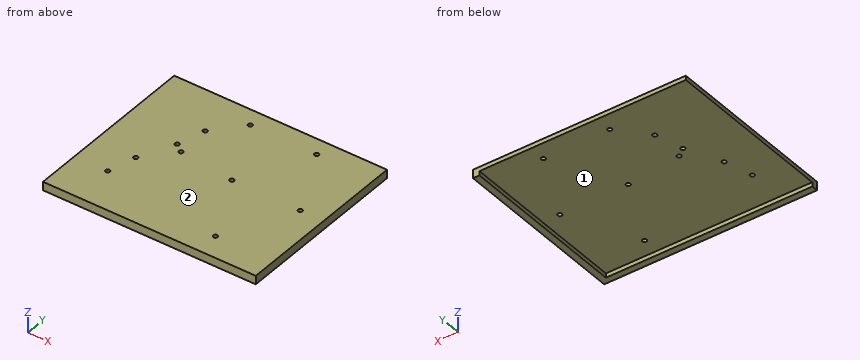
from build123d import *

# Parameters (mm, degrees)
F0_W     = 153.1874
F0_H     = 127
F0_R     = 1.5875
F1_DEPTH = 3.175
F2_DEPTH = 3.175


with BuildPart() as f1:
    # F0 (on Top) → F1 (new body)
    with BuildSketch(Plane.XY):
        Polygon((76.5937, 63.5), (76.5937, -63.5), (-76.5937, -63.5), (-76.5937, -68.2625), (81.3562, -68.2625), (81.3562, 63.5), align=None)
        Rectangle(F0_W, F0_H)
        with Locations((-51.98999, -36.501629)):
            Circle(F0_R, mode=Mode.SUBTRACT)
        with Locations((-46.4312, -15.875)):
            Circle(F0_R, mode=Mode.SUBTRACT)
        with Locations((38.4937, -50.8)):
            Circle(F0_R, mode=Mode.SUBTRACT)
        with Locations((-28.17241, 4.751629)):
            Circle(F0_R, mode=Mode.SUBTRACT)
        with Locations((-34.52749, 9.535871)):
            Circle(F0_R, mode=Mode.SUBTRACT)
        with Locations((-28.9687, 30.1625)):
            Circle(F0_R, mode=Mode.SUBTRACT)
        with Locations((-10.70991, 50.789129)):
            Circle(F0_R, mode=Mode.SUBTRACT)
        with Locations((13.0937, 0)):
            Circle(F0_R, mode=Mode.SUBTRACT)
        with Locations((63.8937, 0)):
            Circle(F0_R, mode=Mode.SUBTRACT)
        with Locations((38.4937, 50.8)):
            Circle(F0_R, mode=Mode.SUBTRACT)
    extrude(amount=F1_DEPTH)

    # F0 (on Top) → F2 (join)
    with BuildSketch(Plane.XY):
        Polygon((76.5937, 63.5), (76.5937, -63.5), (-76.5937, -63.5), (-76.5937, -68.2625), (81.3562, -68.2625), (81.3562, 63.5), align=None)
    extrude(amount=-F2_DEPTH)


solid = f1.part
Input: part model. Units: mm. Frame: model coordinates. Face numbers are marked on the shaded views. A direction names the side the tool comes from. Round coordinates to 2 decimals unless told otherwise and drop trailing zeros. Order: outer loops, then holes, each group sorted by start corner. A loop starts at its lowest first (then second) coordinate and runs counter-clockwise, first axis right, second up. Notation, with made-up numbers: (-26.75, 52.5) - (31.25, 52.5) arc R26 cw to (31.25, 86.5) - close; hole circle Ø11 at (-23, 80). An arc over 180 degrees is marked (long way). Use a Markdown table: item, result.
1. Material intervals for probe 1 along Z at (x, y) = (-1.5, -10.5) (3 decimals); probe 2 along Y at (x, z) = (-1.5, -1.5); probe 3 along X at (y, z) = (30.5, -1), sorted ascending.
Evaluation:
| item | result |
|---|---|
| probe 1 | 0 to 3.175 |
| probe 2 | -68.26 to -63.5 |
| probe 3 | 76.59 to 81.36 |
2. Access query for the marked faces 1 and 2. Directions: +Z, -Z, +X, -X, +Y, -Y. A direction counts if a zero-diameter tool reaches every point of the face in a straight line with its end or side. Return the directions, or none.
Evaluation:
| item | result |
|---|---|
| face 1 | -Z, -X, +Y |
| face 2 | +Z, +X, -X, +Y, -Y |
3. Section A-A on y = 37.5. Return the cut outline in (x, z) (3 decimals).
Evaluation:
| item | result |
|---|---|
| outline | (-76.594, 0) - (76.594, 0) - (76.594, -3.175) - (81.356, -3.175) - (81.356, 3.175) - (-76.594, 3.175) - close |
4. First-contact query: pin 1 (1 mm diameter, centred on x = -28, y = -3.5, fed in from -Z); pin 2 (1.6 mm diameter, centred on y = -21.5, z = -2.5, fed in from -X); pin 3 (2.5 mm diameter, centred on x = -11, z = -1.5, fed in from +Y). Flat tips, straight axial feed; report the tip coordinate or a pass-through.
Evaluation:
| item | result |
|---|---|
| pin 1 | z = 0 |
| pin 2 | x = 76.59 |
| pin 3 | y = -63.5 |
5. Section B-B on x = -2. Return the cut outline in (y, z) (1 decimal), then the cut area to 3 significant figures.
Evaluation:
| item | result |
|---|---|
| outline | (-68.3, -3.2) - (-63.5, -3.2) - (-63.5, 0) - (63.5, 0) - (63.5, 3.2) - (-68.3, 3.2) - close |
| area | 433 mm^2 |
